Design review of the part built by this model. Coordinates are the model's own, in mm. A direction names the side the tool comes from. Round coordinates to 2 decimals unless told otherwise and drop trailing zeros. Order: outer loops, then holes, each group sorted by start corner. A loop starts at its lowest first (then second) coordinate and runs counter-clockwise, first axis right, second up. Notation, with made-up numbers: (-36.75, 35.5) - (-8.75, 35.5) arc R15 ccw to (-8.75, 54.5) - close; hole circle Ø1 at (17.25, 40). An arc over 180 degrees is marked (long way). Write item = value, one per line.
from build123d import *

# Parameters (mm, degrees)
F0_W          = 0.6
F0_H          = 1.8
F1_DEPTH      = 16.4
F1_DEPTH_BACK = 16.4
F0_R          = 10
F0_R_2        = 8
F2_DEPTH      = 15
F2_DEPTH_BACK = 15
F3_W          = 15
F3_H          = 5
F4_DEPTH      = 20
F4_DEPTH_BACK = 20


with BuildPart() as f1:
    # F0 (on Top) → F1 (new body, two sides)
    with BuildSketch(Plane.XY) as f1_sk:
        with Locations((-9, 0)):
            Rectangle(F0_W, F0_H)
    extrude(amount=F1_DEPTH)
    extrude(f1_sk.sketch, amount=-F1_DEPTH_BACK)



with BuildPart() as f1b:
    # F0 (on Top) → F1, piece 2 (new body, two sides)
    with BuildSketch(Plane.XY) as f1_2_sk:
        with Locations((9, 0)):
            Rectangle(F0_W, F0_H)
    extrude(amount=F1_DEPTH)
    extrude(f1_2_sk.sketch, amount=-F1_DEPTH_BACK)


with BuildPart() as f1_1:
    add(f1.part)

    add(f1b.part)  # F2 merges F1b
    # F0 (on Top) → F2 (join, two sides)
    with BuildSketch(Plane.XY) as f2_sk:
        Circle(F0_R)
        with Locations((-9, 0)):
            Rectangle(F0_W, F0_H, mode=Mode.SUBTRACT)
        Circle(F0_R_2, mode=Mode.SUBTRACT)
        with Locations((9, 0)):
            Rectangle(F0_W, F0_H, mode=Mode.SUBTRACT)
    extrude(amount=F2_DEPTH)
    extrude(f2_sk.sketch, amount=-F2_DEPTH_BACK)

    # F3 (on Front) → F4 (cut, two sides)
    with BuildSketch(Plane.XZ) as f4_sk:
        Rectangle(F3_W, F3_H)
    extrude(amount=-F4_DEPTH, mode=Mode.SUBTRACT)
    extrude(f4_sk.sketch, amount=F4_DEPTH_BACK, mode=Mode.SUBTRACT)


solid = f1_1.part
1) To check wall thickness, follow L1, parallel to Z at x = -2.75, y = 8.75; L2, parallel to Y at x = 0, z = 4.5; L3, parallel to Z at x = -8.25, y = -0.75. State the ranges of each line that lie inside material, in increasing order. Write a range as from..to.
Findings:
L1 = -15..-2.5, 2.5..15
L2 = -10..-8, 8..10
L3 = -15..15
2) We need section A-A on x = 0. Write out the cut boundary in (y, z), and give its area (3 significant figures).
Findings:
outline = (-10, -15) - (-8, -15) - (-8, -2.5) - (-10, -2.5) - close; (-10, 2.5) - (-8, 2.5) - (-8, 15) - (-10, 15) - close; (8, -15) - (10, -15) - (10, -2.5) - (8, -2.5) - close; (8, 2.5) - (10, 2.5) - (10, 15) - (8, 15) - close
area = 100 mm^2
3) We need section C-C on y = 4. Write out the cut boundary in (x, z).
Findings:
outline = (-9.17, -15) - (-6.93, -15) - (-6.93, -2.5) - (-7.5, -2.5) - (-7.5, 2.5) - (-6.93, 2.5) - (-6.93, 15) - (-9.17, 15) - close; (6.93, -15) - (9.17, -15) - (9.17, 15) - (6.93, 15) - (6.93, 2.5) - (7.5, 2.5) - (7.5, -2.5) - (6.93, -2.5) - close
4) The part is to be moulded in two halves that separate along Z. For faces 1 (the flat face through (-7.5, 5, 0)), 2 (the flat face through (-8.7, 0, -16)), say which applies: released by +Z, released by -Z, zero draft, split by the parting line, or undercut.
Findings:
face_1 = undercut
face_2 = zero draft
5) Clearance check with flat-ended pins moving along their axes: pin 1 Ø0.7 at (y, z) = (0, 15.5) entering from -X; pin 2 Ø0.5 at (x, z) = (9, 15.5) entering from +Y; pin 3 Ø4 at (x, z) = (-6, 8.5) entering from +Y. State where each tip first meets the part, or that it passes through.
Findings:
pin_1 = -9.3
pin_2 = 0.9
pin_3 = 9.17
6) For faces 3 (the flat face through (-8.7, 0, 16)), 4 (the flat face through (9.3, 0, 16)), 5 (the flat face through (8.7, 0, -16)), 6 (the flat face through (0, -8.2, -2.5)), list the 3-axis set-ups (+Z, -Z, +X, -X, +Y, -Y) from which the entire face can be reached by the end or side of a thin tool; tool diameter is ignored.
Findings:
face_3 = +Z, +Y, -Y
face_4 = +Z, +X, +Y, -Y
face_5 = -Z, +Y, -Y
face_6 = +Y, -Y
7) We need section B-B on z = 1.5. Write out the cut boundary in (x, y).
Findings:
outline = (-7.5, -6.61) - (-7.5, -2.78) arc R8 cw to (-7.5, 2.78) - (-7.5, 6.61) arc R10 ccw to start; (7.5, -6.61) arc R10 ccw to (7.5, 6.61) - (7.5, 2.78) arc R8 cw to (7.5, -2.78) - close
8) We need section D-D on z = -13. Write out the cut boundary in (x, y).
Findings:
outline = circle Ø20 at (0, 0); hole circle Ø16 at (0, 0)
